Can you work these out from the drawing? Everything is in mm from the part's minimum corner. A direction names the side the tool comes from. Give positions to 0.01 mm unless a question says otherwise; leave off trailing zeros. Loops run counter-clockwise (first coordinate to the right, second up) from the corner with the lowest first, then second, coordinate; pieces in that order, holes last. Notation, with made-up numbers: (-31.5, -27.75) - (20.5, -27.75) arc R8 ccw to (20.5, -19.75) - close; hole circle Ø3 at (84, -9.5). An arc over 180 degrees is marked (long way). One line per item, written item: value. Start each with the question number.
Q1. I want a section at C-C (z = 12). Please give me the cut outline in (x, y), then the cut area to 3 significant figures.
Q2. If I drill on line 1 (Z direction, x = 7.75, y = 6) (1 decimal); line 2 (Z direction, x = 13.25, y = 9.5) (1 decimal); line 3 (X direction, y = 0.75, z = 9.75), over which ranges is the centre line in solid material (lowest first)? Write a range as from..to.
Q3. I'm going to push flat-ended pins straight in: P1, Ø1, axis at x = 16, z = 7, coming from the -Y side; P2, Ø1, axis at x = 13, y = 7.5, coming from the -Z side; P3, Ø2, axis at y = 11.5, z = 17, coming from the -X side. Where does each tip first touch, or does it pass through?
Q4. For the marked faces 1, 2, 3 and 4, which set-ups out of +Z, -Z, +X, -X, +Y, -Y let a thin tool reach every point of the face, with its end or its side?
Q5. I want a section at A-A (y = 2.5). Count the separate pieces of the cut face and the enclosed holes in it.
Q6. I want a section at B-B (x = 10). Please give me the cut outline in (y, z).
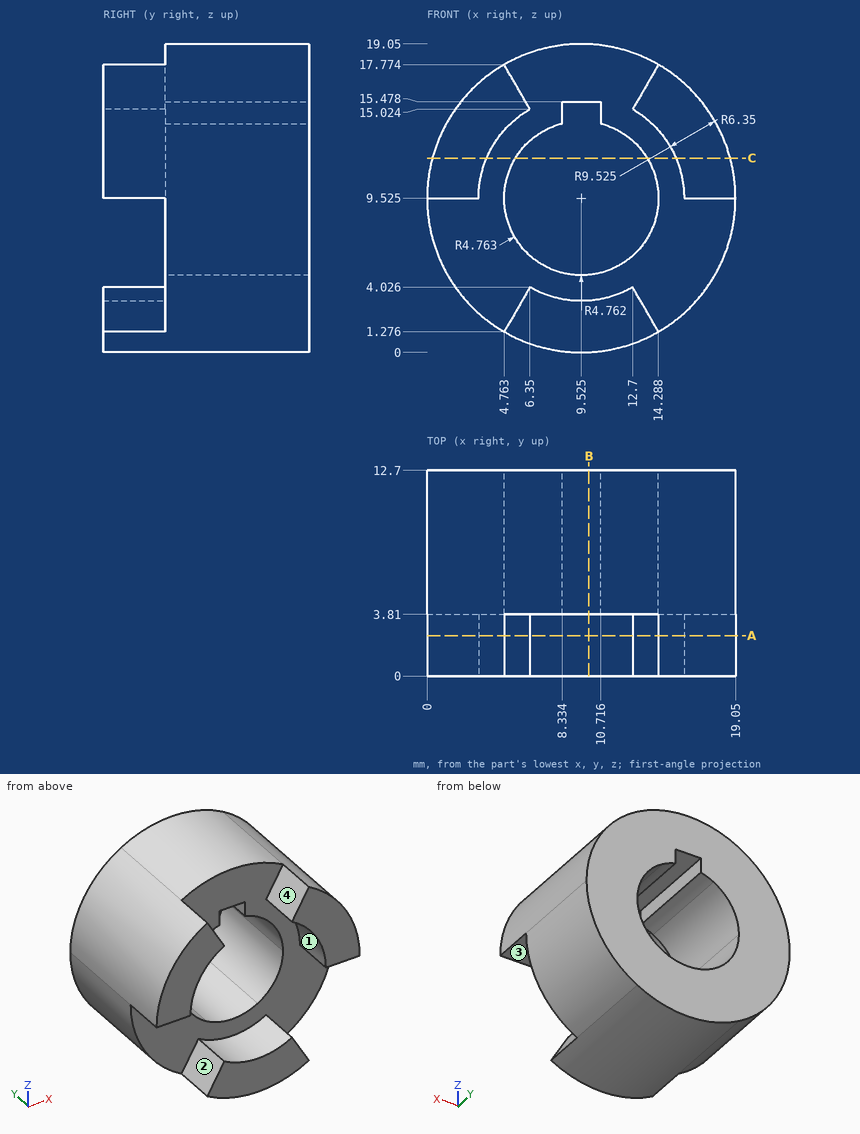
Worked answers:
1. outline: (0.33, 0) - (3.68, 0) - (3.68, 3.81) - (5.46, 3.81) - (5.46, 12.7) - (0.33, 12.7) - close; (13.59, 3.81) - (15.37, 3.81) - (15.37, 0) - (18.72, 0) - (18.72, 12.7) - (13.59, 12.7) - close
1. area: 117 mm²
2. line 1: z = 0.2..5.1, 13.9..18.9
2. line 2: z = 0.8..6.6, 12.5..18.3
2. line 3: x = 0..3.18, 15.87..19.05
3. P1: stops at y = 3.81
3. P2: stops at z = 0.48
3. P3: stops at x = 2.54
4. face 1: -Y
4. face 2: -X, -Y
4. face 3: -Z, +X, -X, -Y
4. face 4: +Z, -Y
5. separate pieces: 3
5. enclosed holes: 0
6. outline: (0, 0.01) - (12.7, 0.01) - (12.7, 4.79) - (3.81, 4.79) - (3.81, 3.19) - (0, 3.19) - close; (3.81, 15.48) - (12.7, 15.48) - (12.7, 19.04) - (3.81, 19.04) - close
